Autodesk Inventor part; units mm, degrees
ref_plane "YZ Plane" through (0, 0, 0) normal (1, 0, 0) x (0, 1, 0)
ref_plane "XZ Plane" through (0, 0, 0) normal (0, 1, 0) x (-1, 0, 0)
ref_plane "XY Plane" through (0, 0, 0) normal (0, 0, 1) x (1, 0, 0)
sketch "Sketch1" plane through (0, 0, 0) normal (0, 0, 1) x (1, 0, 0)
  circle A0 centre (0, 0) radius 16.5
  circle A1 centre (0, 0) radius 18.0545
  dimension "d0" = 33
  dimension "d1" = 1.5545
extrude "Extrusion1" add sketch "Sketch1" along normal blind 5
sketch "Sketch4" plane through (0, 0, 5) normal (0, 0, 1) x (1, 0, 0)
  circle A0 centre (0, 0) radius 12.9
  circle A1 centre (0, 0) radius 14.4627
  dimension "d4" = 25.8
  dimension "d5" = 1.5627
extrude "Extrusion2" add sketch "Sketch4" along normal blind 7.2
sketch "Sketch5" plane through (0, 0, 5) normal (0, 0, 1) x (1, 0, 0)
  circle A0 centre (0, 0) radius 18.0545
  circle A1 centre (0, 0) radius 14.2127
  circle A2 centre (0, 0) radius 18.0545
extrude "Extrusion3" add sketch "Sketch5" along normal blind 4
chamfer "Chamfer2" distance 3.5 angle 45 1 edges at (-18.0545, 0, 9) measured on face at (16.5423, -2.594, 9)
properties part number "850_10_filter_holder_v2"
Source: CAD feature listing. Evaluate the final solid. Frame: model axes, mm. A direction names the side the tool comes from. Give positions to 0.01 mm unless a question says otherwise; leave off trailing zeros. Write each loop counter-clockwise with the first axis right and the second up, starting at its lowest first coordinate (ties: lowest second). Pieces come first, ordered by that corner, then holes. Notation, with made-up numbers: (-33, 8.25) -> (5, 8.25) arc R14 ccw to (5, 25.25) -> close; hole circle Ø4 at (-27.75, 7). An arc over 180 degrees is marked (long way). Write item = value, one per line.
Q1. Mould query, pull axis X, two halves, no side actions, for faces 4 (the face through (8, -15, 0)), 5 (the face through (-1.92, -14.65, 8.78)), 6 (the face through (15.24, 6.32, 2.46)). Classes: +X half, -X half, draft (parallel to the pull), parting line (faces both ways), or undercut.
Here are the results:
face_4 = draft
face_5 = parting line
face_6 = undercut
Q2. Line query: line 1 (Y direction, x = 0, z = 2.4); line 2 (Y direction, x = -0.5, z = 10.75); line 3 (X direction, y = 6, z = 8.5). Output: solid intervals per line, ascending. Write a range as from..to.
Here are the results:
line_1 = -18.05..-16.5, 16.5..18.05
line_2 = -14.45..-12.89, 12.89..14.45
line_3 = -13.81..-11.42, 11.42..13.81
Q3. Cut plane D-D on z = 7.25. Return loops of the section in (x, y), then the cut area to 3 significant figures.
Here are the results:
outline = circle Ø32.61 at (0, 0); hole circle Ø25.8 at (0, 0)
area = 312 mm²
Q4. Cut plane C-C on z = 3.75. Return loops of the section in (x, y).
Here are the results:
outline = circle Ø36.11 at (0, 0); hole circle Ø33 at (0, 0)
Q5. Reachability of faces 1 (the face through (-13, -2, 12.2)), 2 (the face through (7.3, -10.9, 5)), 3 (the face through (13.795, -4.344, 10.578)) from +Z, -Z, +X, -X, +Y, -Y: full face, straight path, thin tool, end or side. Return the list, or none.
Here are the results:
face_1 = +Z, +X, -X, +Y, -Y
face_2 = -Z
face_3 = +Z
Q6. Cut plane A-A on y = 0. Return loops of the section in (x, z), then the cut area to 3 significant figures.
Here are the results:
outline = (-18.05, 0) -> (-16.5, 0) -> (-16.5, 5) -> (-12.9, 5) -> (-12.9, 12.2) -> (-14.46, 12.2) -> (-14.46, 9) -> (-14.55, 9) -> (-18.05, 5.5) -> close; (12.9, 5) -> (16.5, 5) -> (16.5, 0) -> (18.05, 0) -> (18.05, 5.5) -> (14.55, 9) -> (14.46, 9) -> (14.46, 12.2) -> (12.9, 12.2) -> close
area = 54.5 mm²
Q7. First-contact query: pin 1 (12 mm diameter, centred on x = 2, y = -1.5, fed in from -Z); pin 2 (16.5 mm diameter, centred on x = 5, y = -1, fed in from -Z); pin 3 (2 mm diameter, centred on y = 14, z = 7.5, fed in from -X); pin 4 (4 mm diameter, centred on y = 13, z = 2.5, fed in from +X). Flat tips, straight axial feed; report the tip coordinate or a pass-through.
Here are the results:
pin_1 = through
pin_2 = 5
pin_3 = -10.22
pin_4 = 14.32
